Build history of the part. All positions in model axes, mm. Face numbers are marked on the shaded views. Round coordinates to 2 decimals unless told otherwise and drop trailing zeros. Order: outer loops, then holes, each group sorted by start corner. A loop starts at its lowest first (then second) coordinate and runs counter-clockwise, first axis right, second up. Notation, with made-up numbers: M -24,-17.75 L 27,-17.75 A24 cw 27,14.25 Z; hole C -20.75,-35.5 d9. An arc over 180 degrees is marked long. One line per item, written item: value. Start each with the question number.
Item 1: Probe L1, parallel to Z at x = 38.5, y = 0.5; L2, parallel to X at y = -20.5, z = -19; L3, parallel to Z at x = 37, y = -16. List the from-to ranges inside material, lowest first.
Item 2: Band-saw the part on B-B, the plane z = -28.5. Write the cut outline in (x, y), then the cut area to 3 significant figures.
Item 3: Band-saw the part on A-A, the plane x = 23.5. Write the cut outline in (y, z), then the cut area to 3 significant figures.
Item 4: Pin check, flat tips, straight feed: pin 1 (1.8 mm diameter, centred on x = 58.5, z = 2, fed in from -Y); pin 2 (8 mm diameter, centred on x = 8, z = -51, fed in from +Y); pin 3 (5 mm diameter, centred on y = -25.5, z = -20, fed in from -X); pin 4 (3 mm diameter, centred on x = 55, z = 2.5, fed in from +Y). Stop position of each tip, or through.
Item 5: Band-saw the part on D-D, the plane z = -5.5. Write the cut outline in (x, y), then the cut area to 3 significant figures.
Item 6: Two-plate mould, pull along Z, no slides. Class the marked faces 1, 2 and 3: +Z half, -Z half, draft (parallel to the pull), parting line (faces both ways), or undercut.
Item 7: Band-saw the part on C-C, the plane y = -6. Write the cut outline in (x, z), then the cut area to 3 significant figures.
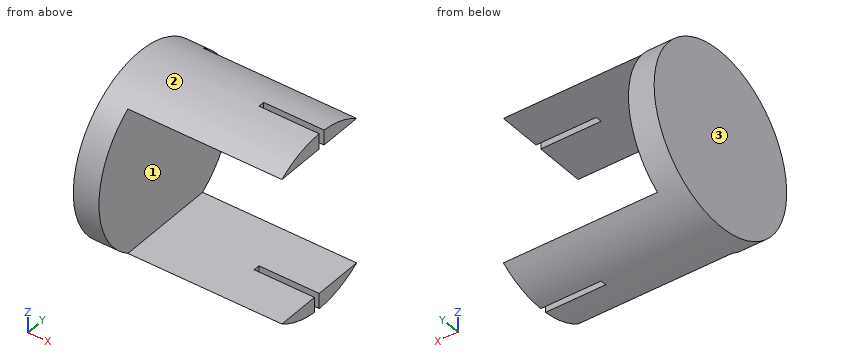
Autodesk Inventor part; units mm, degrees
ref_plane "YZ Plane" through (0, 0, 0) normal (1, 0, 0) x (0, 1, 0)
ref_plane "XZ Plane" through (0, 0, 0) normal (0, 1, 0) x (-1, 0, 0)
ref_plane "XY Plane" through (0, 0, 0) normal (0, 0, 1) x (1, 0, 0)
sketch "Sketch1" plane through (0, 0, 0) normal (1, 0, 0) x (0, 1, 0)
  circle A0 centre (0, -28.5) radius 34.5
  point P0 (0, 0)
extrude "Extrusion1" add sketch "Sketch1" along normal blind 70
sketch "Sketch2" plane through (70, 0, -28.5) normal (1, 0, 0) x (0, 0, -1)
  line L0 (-28.5, 0) -> (-28.5, 19.4422)
  circle A0 centre (0, 0) radius 34.5
  line L1 (-28.5, 0) -> (-28.5, -19.4422)
  line L2 (28.5, 0) -> (28.5, 19.4422)
  line L3 (28.5, 0) -> (28.5, -19.4422)
  arc A1 (-28.5, 19.4422) -> (-28.5, -19.4422) centre (0, 0) ccw
  arc A2 (28.5, -19.4422) -> (28.5, 19.4422) centre (0, 0) ccw
  arc A3 (28.5, 19.4422) -> (-28.5, 19.4422) centre (0, 0) ccw
  arc A4 (-28.5, -19.4422) -> (28.5, -19.4422) centre (0, 0) ccw
extrude "Extrusion2" cut sketch "Sketch2" against normal blind 60 contours L0 A0 L2 L3 L1
sketch "Sketch3" plane through (70, 0, 0) normal (1, 0, 0) x (0, 0, -1)
  line L0 (0, 0) -> (0, 1.25)
  circle A0 centre (28.5, 0) radius 34.5
  line L1 (28.5, 0) -> (28.5, 34.5)
  line L2 (0, 1.25) -> (0, 2.5)
  line L3 (0, -19.4422) -> (0, 19.4422)
  line L4 (0, 2.5) -> (-6.2328, 2.5)
  line L5 (-6.2328, 2.5) -> (-6.2328, 0)
  line L6 (-6.2328, 0) -> (0, 0)
  line L7 (57, 19.4422) -> (57, -19.4422)
  line L8 (57, 0) -> (57, -2.5)
  line L9 (57, -2.5) -> (63.7144, -2.5)
  line L10 (63.7144, -2.5) -> (63.7144, 0)
  line L11 (63.7144, 0) -> (57, 0)
  dimension "d9" = 1.25
  dimension "d10" = 2.5
extrude "Extrusion3" cut sketch "Sketch3" against normal blind 23.5 contours L6 A0 L4 L2 L0 | L6 L5 L4 A0 | L9 L7 L11 A0 | A0 L11 L10 L9
properties part number "Base"
Output:
1. L1: z = -63 to -57, 0 to 6
1. L2: x = 0 to 10
1. L3: z = -59.07 to -57, 0 to 2.07
2. outline: M 0,-34.5 L 10,-34.5 L 10,34.5 L 0,34.5 Z
2. area: 690 mm²
3. outline: M -19.44,-57 A34.5 ccw 19.44,-57 Z; M -19.44,0 L 19.44,0 A34.5 ccw Z
3. area: 317 mm²
4. pin 1: stops at y = -17.72
4. pin 2: stops at y = 29.12
4. pin 3: stops at x = 0
4. pin 4: stops at y = 17.89
5. outline: M 0,-25.71 L 10,-25.71 L 10,25.71 L 0,25.71 Z
5. area: 514 mm²
6. face 1: undercut
6. face 2: parting line
6. face 3: draft
7. outline: M 0,-62.47 L 70,-62.47 L 70,-57 L 10,-57 L 10,0 L 70,0 L 70,5.47 L 0,5.47 Z
7. area: 1,340 mm²
